from build123d import *

# Parameters (mm, degrees)
SKETCH2_W           = 38.1
SKETCH2_H           = 38.1
SKETCH2_W_2         = 25.4
SKETCH2_H_2         = 25.4
BOSS_EXTRUDE1_DEPTH = 609.6
SKETCH3_R           = 4.826
CUT_EXTRUDE1_DEPTH  = 609.6


with BuildPart() as part:
    # Sketch2 → Boss-Extrude1 (new body)
    with BuildSketch(Plane(origin=(0, 0, 0), x_dir=(1, 0, 0), z_dir=(0, 1, 0))):
        Rectangle(SKETCH2_W, SKETCH2_H)
        Rectangle(SKETCH2_W_2, SKETCH2_H_2, mode=Mode.SUBTRACT)
    extrude(amount=BOSS_EXTRUDE1_DEPTH)

    # Sketch3 → Cut-Extrude1 (cut)
    with BuildSketch(Plane.XY.offset(19.05)):
        with Locations((0, 596.9)):
            Circle(SKETCH3_R)
        with Locations((0, 558.8)):
            Circle(SKETCH3_R)
        with Locations((0, 508)):
            Circle(SKETCH3_R)
        with Locations((0, 457.2)):
            Circle(SKETCH3_R)
        with Locations((0, 406.4)):
            Circle(SKETCH3_R)
        with Locations((0, 355.6)):
            Circle(SKETCH3_R)
        with Locations((0, 304.8)):
            Circle(SKETCH3_R)
        with Locations((0, 254)):
            Circle(SKETCH3_R)
        with Locations((0, 203.2)):
            Circle(SKETCH3_R)
        with Locations((0, 152.4)):
            Circle(SKETCH3_R)
        with Locations((0, 101.6)):
            Circle(SKETCH3_R)
        with Locations((0, 50.8)):
            Circle(SKETCH3_R)
    extrude(amount=-CUT_EXTRUDE1_DEPTH, mode=Mode.SUBTRACT)


solid = part.part
CAD build for the part. Positions are in the model's coordinates, mm. A direction names the side the tool comes from. Round coordinates to 2 decimals unless told otherwise and drop trailing zeros. Write each loop counter-clockwise with the first axis right and the second up, starting at its lowest first coordinate (ties: lowest second). Pieces come first, ordered by that corner, then holes.
(1) Slice it at A-A, the plane z = 7.5. Write the cut outline in (x, y), and give its area (3 significant figures).
(2) Slice it at B-B, the plane y = 213. Write the cut outline in (x, z).
(3) Mould opens along Y. For faces 3 (the face through (-13, 609.6, 0)), 4 (the face through (-1.05, 300.09, 15.92)), 5 (the face through (-12.7, 301, 0)) say: pulls with the +Y half, pulls with the -Y half, needs draft (parallel to the pull), parting line crosses it, or undercut.
(4) Probe line 1 along X through (y, z) = (57, 11); line 2 along X through (y, z) = (355.6, -17.5). List the from-to ranges inside material, lowest first.
(5) 3-axis set-ups, long thin cutter, end or side, ignore diameter. For faces 1 (the face through (-1.05, 452.49, -15.83)), 2 (the face through (2.6, 300.5, 12.7)): which of +Z, -Z, +X, -X, +Y, -Y reach the whole face in a straight line?
(6) Drop a flat-ended pin along its axis: P1, Ø7.5, axis at x = 0, y = 203.2, coming from the -Z side. Give the stop position or say it passes through.
From the geometry:
1. outline: (-19.05, 0) - (-12.7, 0) - (-12.7, 609.6) - (-19.05, 609.6) - close; (12.7, 0) - (19.05, 0) - (19.05, 609.6) - (12.7, 609.6) - close
1. area: 7,740 mm2
2. outline: (-19.05, -19.05) - (19.05, -19.05) - (19.05, 19.05) - (-19.05, 19.05) - close; hole (-12.7, -12.7) - (12.7, -12.7) - (12.7, 12.7) - (-12.7, 12.7) - close
3. face 3: pulls with the +Y half
3. face 4: undercut
3. face 5: needs draft
4. line 1: x = -19.05 to -12.7, 12.7 to 19.05
4. line 2: x = -19.05 to -4.83, 4.83 to 19.05
5. face 1: +Z, -Z
5. face 2: +Y, -Y
6. P1: passes through
